Verification items for the finished model (mm, model axes). A direction names the side the tool comes from. Give positions to 0.01 mm unless a question says otherwise; leave off trailing zeros. Loops run counter-clockwise (first coordinate to the right, second up) from the corner with the lowest first, then second, coordinate; pieces in that order, holes last. Notation, with made-up numbers: (34.25, 41) -> (91.25, 41) arc R17 cw to (91.25, 46) -> close; hole circle Ø8 at (85.25, 28.5). An arc over 180 degrees is marked (long way). Answer in a Markdown table with one row per item. Add a question column.
Q1. Release check for a two-part mould opening along X. For faces 1 (the face through (25, 1, -125.714)), 2 (the face through (62.09, 1.52, -117.78)), 3 (the face through (-16.912, 2, -123)), 4 (the face through (-44.43, 1.48, -115.2)) record: pulls with the +X half, pulls with the -X half, needs draft (parallel to the pull), parting line crosses it, or undercut.
Q2. Gauge pin test, flat ends, axial feed: P1, Ø1.5, axis at x = -29, y = 1.5, coming from the +Z side; P2, Ø1.5, axis at y = 2, z = -121.5, coming from the -X side; P3, Ø1.5, axis at x = -20, y = 2, coming from the -Z side. Record the tip position at first contact, or that the pin passes through.
Q3. Material ranges on probe 1 along X at (y, z) = (0.35, -63); probe 2 along X at (y, z) = (0.4, -63.5); probe 3 along Z at (x, y) = (-27, 0.3), recorded low to high.
Q4. Set-up check for faces 5 (the face through (62.48, 1.52, -53.59)), 6 (the face through (-21, 2, -119.714)), 7 (the face through (-32, 1, -50.714)): record each of +Z, -Z, +X, -X, +Y, -Y from which the full face is reachable in a straight line by a thin tool's end or side.
Q5. Section check B-B on z = -33. Enter the section's corners in (x, y), and give its area (3 significant figures).
Q6. Section check C-C on x = 55. Enter the section's corners in (y, z).
Q7. Section check A-A on y = 1.8. Enter the section's corners in (x, z), and give its area (3 significant figures).
Autodesk Inventor part; units mm, degrees
ref_plane "YZ Plane" through (0, 0, 0) normal (1, 0, 0) x (0, 1, 0)
ref_plane "XZ Plane" through (0, 0, 0) normal (0, 1, 0) x (-1, 0, 0)
ref_plane "XY Plane" through (0, 0, 0) normal (0, 0, 1) x (1, 0, 0)
sketch "Sketch8" plane through (0, 0, 0) normal (0, 1, 0) x (-1, 0, 0)
  line L0 (-67.0875, -125.7135) -> (28.9125, -125.7135)
  line L1 (24.9125, -50.7135) -> (13.6258, -19.7036)
  line L2 (39.9125, -50.7135) -> (24.9125, -50.7135)
  line L3 (-67.0875, -49.0809) -> (-67.0875, -125.7135)
  line L4 (13.6258, -19.7036) -> (-67.0875, -49.0809)
  line L5 (39.9125, -50.7135) -> (59.9125, -60.7135)
  line L6 (59.9125, -104.7135) -> (28.9125, -125.7135)
  line L7 (59.9125, -60.7135) -> (59.9125, -104.7135)
  dimension "d129" = 31
  dimension "d131" = 21
  dimension "d147" = 10
  dimension "d154" = 20
  dimension "d155" = 15
  dimension "d162" = 33
  dimension "d163" = 110
  dimension "d164" = 96
  dimension "d183" = 44
extrude "Extrusion9" add sketch "Sketch8" along normal blind 3
sketch "Sketch9" plane through (0, 3, 0) normal (0, 1, 0) x (1, 0, 0)
  circle A0 centre (63.5875, 117.7135) radius 1.5
  circle A1 centre (-56.4125, 102.857) radius 1.5
  circle A2 centre (-56.4125, 62.8766) radius 1.5
  circle A3 centre (-3.7176, 27.5666) radius 1.5
  circle A4 centre (-12.2681, 51.059) radius 1.5
  line L0 (-24.9125, 50.7135) -> (-13.6258, 19.7036)
  line L1 (-13.6258, 19.7036) -> (67.0875, 49.0809)
  line L2 (67.0875, 49.0809) -> (67.0875, 125.7135)
  line L3 (67.0875, 125.7135) -> (-28.9125, 125.7135)
  line L4 (-28.9125, 125.7135) -> (-59.9125, 104.7135)
  line L5 (-59.9125, 104.7135) -> (-59.9125, 60.7135)
  line L6 (-59.9125, 60.7135) -> (-39.9125, 50.7135)
  line L7 (-39.9125, 50.7135) -> (-24.9125, 50.7135)
  line L8 (-56.4125, 102.857) -> (-27.8386, 122.2135) construction
  line L9 (-27.8386, 122.2135) -> (63.5875, 122.2135) construction
  line L10 (63.5875, 122.2135) -> (63.5875, 51.5316) construction
  line L11 (63.5875, 51.5316) -> (-11.534, 24.1896) construction
  line L12 (-11.534, 24.1896) -> (-22.4618, 54.2135) construction
  line L13 (-22.4618, 54.2135) -> (-39.0863, 54.2135) construction
  line L14 (-39.0863, 54.2135) -> (-56.4125, 62.8766) construction
  line L15 (-56.4125, 62.8766) -> (-56.4125, 102.857) construction
  line L16 (-39.9125, 50.7135) -> (-24.9125, 50.7135) construction
  line L17 (-24.9125, 50.7135) -> (-21.6236, 51.9106) construction
  circle A5 centre (63.5875, 52.5809) radius 1.5
  line L18 (-24.9125, 50.7135) -> (-13.6258, 19.7036) construction
  line L19 (-23.5444, 46.9547) -> (-12.2681, 51.059) construction
  circle A6 centre (12.0875, 122.2135) radius 1.5
  point P0 (0, 0)
  dimension "d135" = 3
  dimension "d136" = 3
  dimension "d137" = 3
  dimension "d165" = 3
  dimension "d166" = 3
  dimension "d169" = 3.5
  dimension "d185" = 3
  dimension "d186" = 3.5
  dimension "d187" = 3.5
  dimension "d191" = 12
  dimension "d193" = 4
  dimension "d194" = 12
  dimension "d195" = 4
  dimension "d204" = 8
  dimension "d205" = 3
  dimension "d206" = 55
extrude "Extrusion10" cut sketch "Sketch9" against normal through all contours A0 | A1 | A2 | A3 | A4 | A5 | A6
sketch "Sketch10" plane through (0, 3, 0) normal (0, 1, 0) x (1, 0, 0)
  line L0 (-28.9125, 125.7135) -> (-59.9125, 104.7135)
  line L1 (67.0875, 125.7135) -> (-28.9125, 125.7135)
  line L2 (-24.9125, 125.7135) -> (-16.9125, 125.7135)
  line L3 (-16.9125, 125.7135) -> (-16.9125, 119.7135)
  line L4 (-16.9125, 119.7135) -> (-24.9125, 119.7135)
  line L5 (-24.9125, 119.7135) -> (-24.9125, 125.7135)
  point P0 (-17.0619, -65.3949)
  dimension "d179" = 4
  dimension "d180" = 6
  dimension "d181" = 8
extrude "Extrusion11" cut sketch "Sketch10" against normal through all
fillet "Fillet1" radius 2 1 edges at (-39.9125, 1.5, -50.7135)
fillet "Fillet2" radius 2 1 edges at (-59.9125, 1.5, -60.7135)
fillet "Fillet3" radius 2 1 edges at (-59.9125, 1.5, -104.7135)
fillet "Fillet4" radius 2 1 edges at (-28.9125, 1.5, -125.7135)
fillet "Fillet5" radius 2 1 edges at (67.0875, 1.5, -125.7135)
fillet "Fillet6" radius 2 1 edges at (67.0875, 1.5, -49.0809)
properties part number "k2_base"
Taken from the geometry:
| question | item | result |
|---|---|---|
| 1 | face 1 | needs draft |
| 1 | face 2 | undercut |
| 1 | face 3 | undercut |
| 1 | face 4 | pulls with the -X half |
| 2 | P1 | stops at z = -50.71 |
| 2 | P2 | stops at x = -36.24 |
| 2 | P3 | stops at z = -119.71 |
| 3 | probe 1 | x = -59.91 to -57.91, -54.92 to 67.09 |
| 3 | probe 2 | x = -59.91 to -57.78, -55.05 to 67.09 |
| 3 | probe 3 | z = -125.71 to -50.71 |
| 4 | face 5 | +Y, -Y |
| 4 | face 6 | -Z, +Y, -Y |
| 4 | face 7 | +Z, -X, +Y, -Y |
| 5 | outline | (-18.47, 0) -> (22.91, 0) -> (22.91, 3) -> (-18.47, 3) -> close |
| 5 | area | 124 mm² |
| 6 | outline | (0, -125.71) -> (3, -125.71) -> (3, -44.68) -> (0, -44.68) -> close |
| 7 | outline | (-59.91, -103.65) arc R2 ccw to (-59.03, -105.31) -> (-29.42, -125.37) arc R2 ccw to (-28.3, -125.71) -> (-24.91, -125.71) -> (-24.91, -119.71) -> (-16.91, -119.71) -> (-16.91, -125.71) -> (65.09, -125.71) arc R2 ccw to (67.09, -123.71) -> (67.09, -50.48) arc R2 ccw to (65.77, -48.6) -> (-13.63, -19.7) -> (-24.91, -50.71) -> (-39.44, -50.71) arc R2 ccw to (-40.33, -50.92) -> (-58.81, -60.16) arc R2 ccw to (-59.91, -61.95) -> close; hole circle Ø3 at (-56.41, -102.86); hole circle Ø3 at (-56.41, -62.88); hole circle Ø3 at (-12.27, -51.06); hole circle Ø3 at (-3.72, -27.57); hole circle Ø3 at (12.09, -122.21); hole circle Ø3 at (63.59, -117.71); hole circle Ø3 at (63.59, -52.58) |
| 7 | area | 10,500 mm² |
